Build history of the part. All positions in model axes, mm. A direction names the side the tool comes from. Round coordinates to 2 decimals unless told otherwise and drop trailing zeros. Loops run counter-clockwise (first coordinate to the right, second up) from the corner with the lowest first, then second, coordinate; pieces in that order, holes last. Notation, with made-up numbers: (22, 56) - (28, 56) arc R17 cw to (28, 63) - close; hole circle Ø2 at (88, 32). An arc over 180 degrees is marked (long way). Answer as CSV lines item,"result". Start each with the question number.
```python
from build123d import *

# Parameters (mm, degrees)
SKIZZE1_R                       = 8.55
SKIZZE1_W                       = 3
SKIZZE1_H                       = 10
AUFSATZ_LINEAR_AUSTRAGEN1_DEPTH = 4
SKIZZE2_R                       = 10.55
SKIZZE2_W                       = 3
SKIZZE2_H                       = 10
AUFSATZ_LINEAR_AUSTRAGEN2_DEPTH = 7
SKIZZE3_R                       = 7.5
SKIZZE3_W                       = 3
SKIZZE3_H                       = 10
AUFSATZ_LINEAR_AUSTRAGEN3_DEPTH = 2.2
FASE1_SIZE                      = 0.5
SKIZZE4_R                       = 1.8
SCHNITT_LINEAR_AUSTRAGEN1_DEPTH = 10


with BuildPart() as part:
    # Skizze1 → Aufsatz-Linear austragen1 (new body)
    with BuildSketch(Plane(origin=(0, 0, 0), x_dir=(1, 0, 0), z_dir=(0, 1, 0))):
        Circle(SKIZZE1_R)
        Rectangle(SKIZZE1_W, SKIZZE1_H, mode=Mode.SUBTRACT)
    extrude(amount=AUFSATZ_LINEAR_AUSTRAGEN1_DEPTH)

    # Skizze2 → Aufsatz-Linear austragen2 (add)
    with BuildSketch(Plane(origin=(0, 4, 0), x_dir=(1, 0, 0), z_dir=(0, 1, 0))):
        Circle(SKIZZE2_R)
        Rectangle(SKIZZE2_W, SKIZZE2_H, mode=Mode.SUBTRACT)
    extrude(amount=AUFSATZ_LINEAR_AUSTRAGEN2_DEPTH)

    # Skizze3 → Aufsatz-Linear austragen3 (add)
    with BuildSketch(Plane.XZ):
        Circle(SKIZZE3_R)
        Rectangle(SKIZZE3_W, SKIZZE3_H, mode=Mode.SUBTRACT)
    extrude(amount=AUFSATZ_LINEAR_AUSTRAGEN3_DEPTH)

    # Fase1
    fase1_edges = [part.edges().sort_by_distance(p)[0] for p in [
        (-8.55, 0, 0),
    ]]
    chamfer(fase1_edges, length=FASE1_SIZE)

    # Skizze4 → Schnitt-Linear austragen1 (cut)
    with BuildSketch(Plane.XZ.offset(-11)):
        with Locations((-5, 0)):
            Circle(SKIZZE4_R)
        with Locations((5, 0)):
            Circle(SKIZZE4_R)
    extrude(amount=SCHNITT_LINEAR_AUSTRAGEN1_DEPTH, mode=Mode.SUBTRACT)


solid = part.part
```
Q1. Two-plate mould, pull along X, no slides. Class faces 5 (the cylindrical face through (10.063, 7.451, -3.169)), 6 (the flat face through (0, 4, 5)), 7 (the flat face through (2, 11, 0)): released by +X, released by -X, zero draft, split by the parting line, or undercut.
Q2. Band-saw the part on A-A, the plane y = 2. List the corners of the cut face in (x, z).
Q3. Tool access for faces 1 (the cylindrical face through (8.155, 2.226, -2.568)), 2 (the cylindrical face through (6.717, 6.07, 0.541)), 3 (the flat face through (2, -2.2, 0)), 4 (the flat face through (-1.5, 4, 0)): list every direction of +Z, -Z, +X, -X, +Y, -Y with a clear straight run to the whole face (end or side of a thin tool).
Q4. Band-saw the part on B-B, the plane x = 0. List the corners of the cut face in (y, z).
Q5. Pin check, flat tips, straight feed: pin 1 Ø5 at (y, z) = (5.5, 5.5) entering from -X; pin 2 Ø3.5 at (x, y) = (0.5, 1.5) entering from -Z; pin 3 Ø2 at (x, y) = (8.5, 5) entering from -Z. Stop position of each tip, or through.
Q6. Band-saw the part on C-C, the plane z = 0. List the corners of the cut face in (x, y).
Q7. Wall check: probe 1 along X at (y, z) = (5.5, -0.5); probe 2 along X at (y, z) = (3.75, 1); probe 3 along Z at (x, y) = (5, 7.25). Give the ranges that are in metal, low to high. Write a range as [from, to].
Reported:
1,face 5,"split by the parting line"
1,face 6,"undercut"
1,face 7,"zero draft"
2,outline,"circle Ø17.1 at (0, 0); hole circle Ø3.6 at (-5, 0); hole (-1.5, -5) - (1.5, -5) - (1.5, 5) - (-1.5, 5) - close; hole circle Ø3.6 at (5, 0)"
3,face 1,"-Y"
3,face 2,"+Y"
3,face 3,"+Z, -Z, +X, -X, -Y"
3,face 4,"+Y, -Y"
4,outline,"(-2.2, -7.5) - (0, -7.5) - (0, -8.05) - (0.5, -8.55) - (4, -8.55) - (4, -10.55) - (11, -10.55) - (11, -5) - (-2.2, -5) - close; (-2.2, 5) - (11, 5) - (11, 10.55) - (4, 10.55) - (4, 8.55) - (0.5, 8.55) - (0, 8.05) - (0, 7.5) - (-2.2, 7.5) - close"
5,pin 1,"stops at x = -10.11"
5,pin 2,"stops at z = -8.55"
5,pin 3,"stops at z = -7.42"
6,outline,"(-10.55, 4) - (-8.55, 4) - (-8.55, 0.5) - (-8.05, 0) - (-7.5, 0) - (-7.5, -2.2) - (-1.5, -2.2) - (-1.5, 11) - (-3.2, 11) - (-3.2, 1) - (-6.8, 1) - (-6.8, 11) - (-10.55, 11) - close; (1.5, -2.2) - (7.5, -2.2) - (7.5, 0) - (8.05, 0) - (8.55, 0.5) - (8.55, 4) - (10.55, 4) - (10.55, 11) - (6.8, 11) - (6.8, 1) - (3.2, 1) - (3.2, 11) - (1.5, 11) - close"
7,probe 1,"x = [-10.54, -6.73], [-3.27, -1.5], [1.5, 3.27], [6.73, 10.54]"
7,probe 2,"x = [-8.49, -6.5], [-3.5, -1.5], [1.5, 3.5], [6.5, 8.49]"
7,probe 3,"z = [-9.29, -1.8], [1.8, 9.29]"
